Read the model definition and answer for the solid it produces. Units are mm, in the model's axes. Face numbers are marked on the shaded views. Give positions to 0.01 mm unless a question says otherwise; leave off trailing zeros. Loops run counter-clockwise (first coordinate to the right, second up) from the corner with the lowest first, then second, coordinate; pieces in that order, holes last.
(1) Determine the mould class of the marked faces 1, 2, 3 and 4 for opening direction Y: pulls with the +Y half, pulls with the -Y half, needs draft (parallel to the pull), parting line crosses it, or undercut.
(2) Straight lines are drawn through the part: probe 1 along Y at (x, z) = (48, 6); probe 2 along Z at (x, y) = (40, 2); probe 3 along Y at (x, z) = (35, 4.75). For each, find the intervals that lie inside material, in ascending order.
(3) Each of these flat-tipped pins is pushed along its axis until it touches: P1, Ø2, axis at x = 10, z = 4, coming from the -Y side; P2, Ø3, axis at x = 40, z = 4, coming from the -Y side (3 decimals); P3, Ø3, axis at y = 43, z = 4.5, coming from the -X side. Where does it stop, or does it pass through?
(4) Find section A-A, the plane x = 35. Write down the section's boundary in (y, z).
(5) Find section D-D, the plane y = 40. Write down the section's boundary in (x, z), then the cut area to 3 significant figures.
(6) Find section B-B, the plane y = 21.5. Write down the section's boundary in (x, z), then the cut area to 3 significant figures.
(7) Find section C-C, the plane z = 6.25. Write down the section's boundary in (x, y).
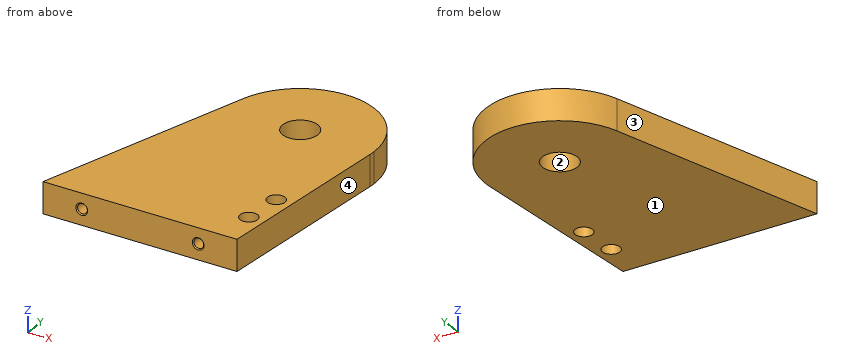
```python
from build123d import *

# Parameters (mm, degrees)
EXTRUDE_1_DEPTH              = 8
HOLE_WIZARD_M4_1_D           = 4.5
HOLE_WIZARD_M3_1_D           = 2.5
HOLE_WIZARD_M3_1_DEPTH       = 8.5
HOLE_WIZARD_M3_1_CSINK_D     = 3.05
HOLE_WIZARD_M3_1_CSINK_ANGLE = 90
HOLE_WIZARD_M3_1_TIP         = 0.751075774
HOLE_WIZARD_M8_1_D           = 9


with BuildPart() as part:
    # 스케치1 → 보스-돌출1 (new body)
    with BuildSketch(Plane.XY):
        with BuildLine():
            Line((16.816107383, 55.508724832), (0, 0))
            Line((0, 0), (50, 0))
            Line((50, 0), (53.937590447, 48.461277134))
            ThreePointArc((53.937590447, 48.461277134), (31.456182162, 31.333416083), (16.816107383, 55.508724832))
        make_face()
        with BuildLine():
            ThreePointArc((54, 50), (37.784424561, 68.794865785), (16.816107383, 55.508724832))
            ThreePointArc((16.816107383, 55.508724832), (31.456182162, 31.333416083), (53.937590447, 48.461277134))
            ThreePointArc((53.937590447, 48.461277134), (53.9843912, 49.230006005), (54, 50))
        make_face()
    extrude(amount=EXTRUDE_1_DEPTH)

    # M4 여유 구멍1 (through all)
    with Locations(Plane.XY.offset(8)):
        with Locations((46.799340892, 10), (47.609195032, 19.967152867)):
            Hole(HOLE_WIZARD_M4_1_D / 2)

    # M3 나사 구멍1
    with Locations(Plane(origin=(0, 0, 0), x_dir=(-1, 0, 0), z_dir=(0, -1, 0))):
        with Locations((-10, -4), (-40, -4)):
            CounterSinkHole(HOLE_WIZARD_M3_1_D / 2, HOLE_WIZARD_M3_1_CSINK_D / 2, depth=HOLE_WIZARD_M3_1_DEPTH, counter_sink_angle=HOLE_WIZARD_M3_1_CSINK_ANGLE)
            with Locations((0, 0, -(HOLE_WIZARD_M3_1_DEPTH + HOLE_WIZARD_M3_1_TIP / 2))):  # 118° drill point
                Cone(0, HOLE_WIZARD_M3_1_D / 2, HOLE_WIZARD_M3_1_TIP, mode=Mode.SUBTRACT)

    # M8 여유 구멍1 (through all)
    with Locations(Plane(origin=(0, 0, 0), x_dir=(-1, 0, 0), z_dir=(0, 0, -1))):
        with Locations((-35, 50)):
            Hole(HOLE_WIZARD_M8_1_D / 2)


solid = part.part
```
Entries:
1. face 1: needs draft
1. face 2: undercut
1. face 3: pulls with the +Y half
1. face 4: pulls with the -Y half
2. probe 1: y = 0 to 8.1, 11.9 to 17.75, 22.18 to 63.86
2. probe 2: z = 0 to 2.75, 5.25 to 8
2. probe 3: y = 0 to 45.5, 54.5 to 69
3. P1: stops at y = 8.65
3. P2: stops at y = 0.025
3. P3: stops at x = 12.57
4. outline: (0, 0) - (45.5, 0) - (45.5, 8) - (0, 8) - close; (54.5, 0) - (69, 0) - (69, 8) - (54.5, 8) - close
5. outline: (12.12, 0) - (53.25, 0) - (53.25, 8) - (12.12, 8) - close
5. area: 329 mm2
6. outline: (6.51, 0) - (45.96, 0) - (45.96, 8) - (6.51, 8) - close; (49.26, 0) - (51.75, 0) - (51.75, 8) - (49.26, 8) - close
6. area: 336 mm2
7. outline: (0, 0) - (50, 0) - (53.94, 48.46) arc R19 ccw to (16.82, 55.51) - close; hole circle Ø9 at (35, 50); hole circle Ø4.5 at (46.8, 10); hole circle Ø4.5 at (47.61, 19.97)
